Check sheet for the drawn part. Datum: minimum x, y, z corner. Units: mm. Give positions to 0.01 mm unless a question says otherwise; leave off trailing zeros. Write each loop counter-clockwise with the first axis right and the second up, starting at its lowest first coordinate (ties: lowest second). Pieces come first, ordered by that corner, then holes. Notation, with made-up numbers: M 47.5,67.5 L 73.5,67.5 A21 ccw 73.5,105.5 Z; hole C 2,70 d4. An arc over 180 degrees is marked long. Use CSV: the item, a comma, the result in double quotes. Start each with the question number.
1. Depth check by flat-ended pin: P1, Ø3, axis at y = 2.5, z = 47.5, coming from the -X side (1 decimal); P2, Ø3, axis at x = 60.325, z = 15.24, coming from the +Y side; P3, Ø3, axis at x = 22.5, y = 5, coming from the -Z side (1 decimal); P4, Ø2, axis at x = 41.5, y = 1, coming from the -Z side (1 decimal). Enter the tip coordinate at first touch or a pass-through.
2. Cross-section at A-A, the plane z = 45. Enter the section's corners in (x, y).
3. Cross-section at B-B, the plane y = 2.5. State how many separate pieces and enclosed holes the cut face has, and give its area (3 significant figures).
4. Cross-section at C-C, the plane x = 38.1. Enter the section's corners in (y, z), and give its area (3 significant figures).
5. Scan lines: line 1 (Z direction, x = 27.5, y = 2) (1 decimal); line 2 (X direction, y = 2.25, z = 39) (1 decimal); line 3 (Z direction, x = 10, y = 2.5) (1 decimal). Record each from-to range of solid material in increasing order.
6. Cross-section at D-D, the plane z = 15.24. Enter the section's corners in (x, y).
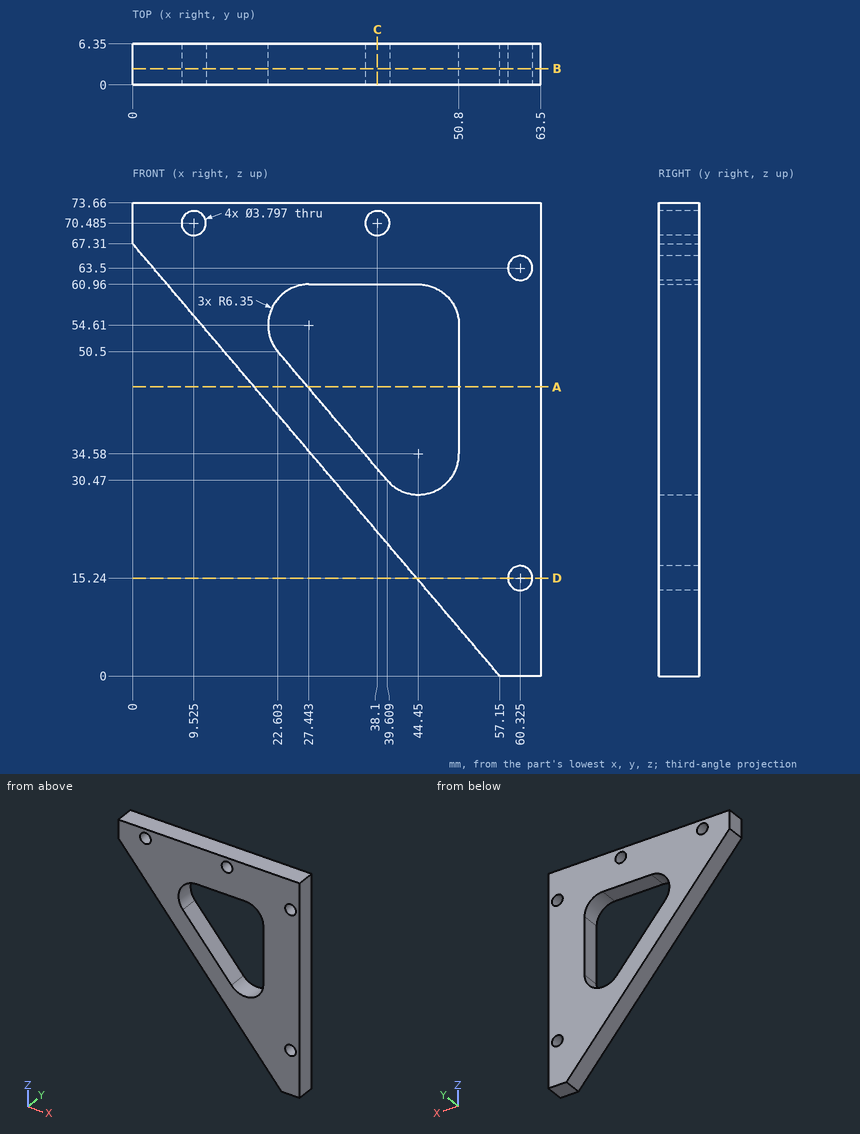
Worked answers:
1,P1,"stops at x = 15.5"
1,P2,"passes through"
1,P3,"stops at z = 39"
1,P4,"stops at z = 17.3"
2,outline,"M 18.94,0 L 27.27,0 L 27.27,6.35 L 18.94,6.35 Z; M 50.8,0 L 63.5,0 L 63.5,6.35 L 50.8,6.35 Z"
3,separate pieces,"1"
3,enclosed holes,"5"
3,area,"2,010 mm^2"
4,outline,"M 0,22.44 L 6.35,22.44 L 6.35,32.25 L 0,32.25 Z; M 0,60.96 L 6.35,60.96 L 6.35,68.59 L 0,68.59 Z; M 0,72.38 L 6.35,72.38 L 6.35,73.66 L 0,73.66 Z"
4,area,"119 mm^2"
5,line 1,"z = 34.9 to 44.7, 61 to 73.7"
5,line 2,"x = 24 to 32.4, 50.8 to 63.5"
5,line 3,"z = 55.5 to 68.6, 72.3 to 73.7"
6,outline,"M 44.21,0 L 58.43,0 L 58.43,6.35 L 44.21,6.35 Z; M 62.22,0 L 63.5,0 L 63.5,6.35 L 62.22,6.35 Z"
